```python
from build123d import *

# Parameters (mm, degrees)
BOSS_EXTRUDE4_DEPTH = 20
BOSS_EXTRUDE7_START = -20
BOSS_EXTRUDE7_DEPTH = 20
SKETCH12_R          = 1.65
CUT_EXTRUDE1_DEPTH  = 177.068006068


with BuildPart() as part:
    # Sketch5 → Boss-Extrude4 (new body)
    with BuildSketch(Plane.XY):
        with BuildLine():
            Line((0, 0), (0, 167.041245738))
            ThreePointArc((0, 167.041245738), (-1.523254023, 168.9835931), (-3.772713274, 167.967252028))
            ThreePointArc((-3.772713274, 167.967252028), (-34.542452011, 86.476422979), (-45, 0))
            Line((-45, 0), (0, 0))
        make_face()
        with BuildLine():
            Line((-1.6, 10), (-40.860610891, 10))
            ThreePointArc((-40.860610891, 10), (-30.458147518, 86.332115465), (-4, 158.683822602))
            ThreePointArc((-4, 158.683822602), (-2.577933762, 159.356407939), (-1.6, 158.124219244))
            Line((-1.6, 158.124219244), (-1.6, 10))
        make_face(mode=Mode.SUBTRACT)
    extrude(amount=BOSS_EXTRUDE4_DEPTH)

    # Sketch11 → Boss-Extrude7 (add)
    with BuildSketch(Plane.XY.offset(20).offset(BOSS_EXTRUDE7_START)):
        with BuildLine():
            ThreePointArc((-40.61576824, 16.6), (-40.651926046, 15.800039355), (-40.686298284, 15))
            Line((-40.686298284, 15), (-1.6, 15))
            Line((-1.6, 15), (-1.6, 16.6))
            Line((-1.6, 16.6), (-40.61576824, 16.6))
        make_face()
        with BuildLine():
            ThreePointArc((-39.849641566, 28.707538392), (-39.912786801, 27.909744506), (-39.974152323, 27.111811753))
            Line((-39.974152323, 27.111811753), (-1.6, 23.078525819))
            Line((-1.6, 23.078525819), (-1.6, 24.687339066))
            Line((-1.6, 24.687339066), (-39.849641566, 28.707538392))
        make_face()
        with BuildLine():
            ThreePointArc((-38.660345477, 40.906700159), (-38.751098874, 40.10802838), (-38.840062688, 39.30915528))
            Line((-38.840062688, 39.30915528), (-1.6, 31.393535598))
            Line((-1.6, 31.393535598), (-1.6, 33.02928055))
            Line((-1.6, 33.02928055), (-38.660345477, 40.906700159))
        make_face()
        with BuildLine():
            ThreePointArc((-37.013521794, 53.335050155), (-37.133222882, 52.532613088), (-37.251109088, 51.729907388))
            Line((-37.251109088, 51.729907388), (-1.6, 40.146159853))
            Line((-1.6, 40.146159853), (-1.6, 41.828499411))
            Line((-1.6, 41.828499411), (-37.013521794, 53.335050155))
        make_face()
        with BuildLine():
            ThreePointArc((-34.852060307, 66.133887827), (-35.002794049, 65.325048554), (-35.151672531, 64.515865738))
            Line((-35.151672531, 64.515865738), (-1.6, 49.577698687))
            Line((-1.6, 49.577698687), (-1.6, 51.329116733))
            Line((-1.6, 51.329116733), (-34.852060307, 66.133887827))
        make_face()
        with BuildLine():
            ThreePointArc((-32.092292656, 79.450787546), (-32.27693125, 78.633291388), (-32.45965971, 77.815366152))
            Line((-32.45965971, 77.815366152), (-1.6, 59.998533312))
            Line((-1.6, 59.998533312), (-1.6, 61.846054173))
            Line((-1.6, 61.846054173), (-32.092292656, 79.450787546))
        make_face()
        with BuildLine():
            ThreePointArc((-28.966005847, 92.142511062), (-29.146660506, 91.459980039), (-29.325971671, 90.77709483))
            Line((-29.325971671, 90.77709483), (-1.6, 69.30954071))
            Line((-1.6, 69.30954071), (-1.6, 70.953669837))
            Line((-1.6, 70.953669837), (-28.966005847, 92.142511062))
        make_face()
        with BuildLine():
            ThreePointArc((-25.415771616, 104.592932273), (-25.62575353, 103.901436527), (-25.834342161, 103.209519225))
            Line((-25.834342161, 103.209519225), (-1.6, 80.807713123))
            Line((-1.6, 80.807713123), (-1.6, 82.578045531))
            Line((-1.6, 82.578045531), (-25.415771616, 104.592932273))
        make_face()
        with BuildLine():
            ThreePointArc((-21.12443405, 117.757312491), (-21.366950886, 117.057023911), (-21.608020686, 116.356235882))
            Line((-21.608020686, 116.356235882), (-1.6, 94.329309417))
            Line((-1.6, 94.329309417), (-1.6, 96.262768885))
            Line((-1.6, 96.262768885), (-21.12443405, 117.757312491))
        make_face()
        with BuildLine():
            ThreePointArc((-15.938835517, 131.737298585), (-16.21749388, 131.029204139), (-16.49464978, 130.320520265))
            Line((-16.49464978, 130.320520265), (-1.6, 110.733232757))
            Line((-1.6, 110.733232757), (-1.6, 112.880937546))
            Line((-1.6, 112.880937546), (-15.938835517, 131.737298585))
        make_face()
        with BuildLine():
            ThreePointArc((-9.669507991, 146.627994836), (-9.988229593, 145.91414681), (-10.30539498, 145.199605992))
            Line((-10.30539498, 145.199605992), (-1.6, 131.402518814))
            Line((-1.6, 131.402518814), (-1.6, 133.83871813))
            Line((-1.6, 133.83871813), (-9.669507991, 146.627994836))
        make_face()
    extrude(amount=BOSS_EXTRUDE7_DEPTH)

    # Sketch12 → Cut-Extrude1 (cut, through all)
    with BuildSketch(Plane.XY.offset(20)):
        with Locations((-40, 5)):
            Circle(SKETCH12_R)
        with Locations((-22.5, 5)):
            Circle(SKETCH12_R)
        with Locations((-5, 5)):
            Circle(SKETCH12_R)
    extrude(amount=-CUT_EXTRUDE1_DEPTH, mode=Mode.SUBTRACT)


solid = part.part
```
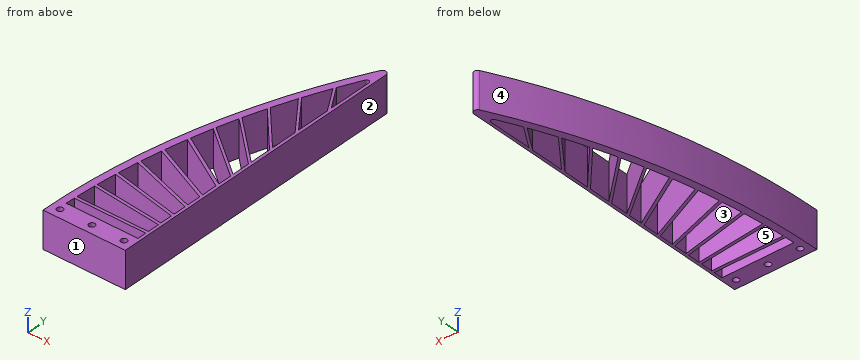
The listing builds one solid part. Answer for the finished solid, in the listing's coordinates (mm). Face numbers are marked on the shaded views. A direction names the side the tool comes from. Give positions to 0.01 mm unless a question says otherwise; leave off trailing zeros. Order: outer loops, then holes, each group sorted by start corner. A loop starts at its lowest first (then second) coordinate and runs counter-clockwise, first axis right, second up. Notation, with made-up numbers: (57.25, 25.5) -> (98.25, 25.5) arc R34 ccw to (98.25, 58.5) -> close; hole circle Ø8 at (26.25, 21.25). An arc over 180 degrees is marked (long way). Answer as a JSON object with one key per item and string values. Group by question number.
Item 1: The part is cut by section C-C on y = 5. Write down the section's boundary in (x, z), and give its area (3 significant figures).
Item 2: Determine the mould class of the marked faces 1, 2 and 3 for opening direction X: pulls with the +X half, pulls with the -X half, needs draft (parallel to the pull), parting line crosses it, or undercut.
Item 3: The part is cut by section A-A on y = 85. Write down the section's boundary in (x, z), and give its area (3 significant figures).
Item 4: Flat-ended cylindrical pins translate along their axes: pin 1 (7.5 mm diameter, centred on y = 28, z = 8, fed in from -X); pin 2 (3 mm diameter, centred on x = -17, z = 14, fed in from +Y); pin 3 (1.9 mm diameter, centred on y = 20, z = 10, fed in from -X). Find the tip coordinate at first contact, or state that the pin passes through.
Item 5: A tool of negligible diameter and unlimited length cuts with its end or side. For the marked faces 4 and 5, from which of +Z, -Z, +X, -X, +Y, -Y can it reach the whole face along a straight path? Write none if from no direction.
Item 6: Consider L1, parallel to X at y = 88.5, z = 1.5; L2, parallel to X at y = 94, z = 14.25; L3, parallel to X at y = 82.5, z = 4.75. Determine where each line is inside the solid, lowest interval first. Write a range as from..to.
Item 7: The part is cut by section B-B on z = 10.75. Give the number of separate pieces and of enclosed holes in the cut face, and give its area (3 significant figures).
Result set:
{
 "1": {"outline": "(-44.97, 0) -> (-41.65, 0) -> (-41.65, 20) -> (-44.97, 20) -> close; (-38.35, 0) -> (-24.15, 0) -> (-24.15, 20) -> (-38.35, 20) -> close; (-20.85, 0) -> (-6.65, 0) -> (-6.65, 20) -> (-20.85, 20) -> close; (-3.35, 0) -> (0, 0) -> (0, 20) -> (-3.35, 20) -> close", "area": "701 mm²"},
 "2": {"face 1": "needs draft", "face 2": "pulls with the +X half", "face 3": "undercut"},
 "3": {"outline": "(-34.9, 0) -> (-30.79, 0) -> (-30.79, 20) -> (-34.9, 20) -> close; (-21.86, 0) -> (-19.74, 0) -> (-19.74, 20) -> (-21.86, 20) -> close; (-6.14, 0) -> (-4.22, 0) -> (-4.22, 20) -> (-6.14, 20) -> close; (-1.6, 0) -> (0, 0) -> (0, 20) -> (-1.6, 20) -> close", "area": "195 mm²"},
 "4": {"pin 1": "x = -44.19", "pin 2": "y = 143.3", "pin 3": "x = -44.5"},
 "5": {"face 4": "+Z, -Z, -X, +Y", "face 5": "+Z, -Z"},
 "6": {"L1": "-34.04..-29.91, -26.39..-24.26, -9.92..-8.01, -1.6..0", "L2": "-32.61..-28.47, -15.87..-13.96, -1.6..0", "L3": "-35.49..-31.39, -18.64..-16.51, -3.43..0"},
 "7": {"separate pieces": "1", "enclosed holes": "15", "area": "1,880 mm²"}
}
